Autodesk Inventor part; units mm, degrees
ref_plane "YZ Plane" through (0, 0, 0) normal (1, 0, 0) x (0, 1, 0)
ref_plane "XZ Plane" through (0, 0, 0) normal (0, 1, 0) x (-1, 0, 0)
ref_plane "XY Plane" through (0, 0, 0) normal (0, 0, 1) x (1, 0, 0)
sketch "Sketch1" plane through (0, 0, 0) normal (0, 0, 1) x (1, 0, 0)
  line L0 (0, 0) -> (25, 0)
  line L1 (25, 0) -> (25, 55.5)
  line L2 (25, 55.5) -> (0, 55.5)
  line L3 (0, 55.5) -> (0, 0)
  dimension "d0" = 25
  dimension "d1" = 55.5
extrude "Extrusion1" add sketch "Sketch1" along normal blind 3
sketch "Sketch2" plane through (0, 0, 3) normal (0, 0, 1) x (1, 0, 0)
  line L0 (0, 55.5) -> (0, 0)
  line L1 (25, 55.5) -> (0, 55.5)
  line L2 (0, 0) -> (3, 0)
  line L3 (3, 0) -> (3, 55.5)
  line L4 (3, 55.5) -> (0, 55.5)
  line L5 (0, 55.5) -> (0, 0)
  dimension "d4" = 3
extrude "Extrusion2" cut sketch "Sketch2" against normal through all
sketch "Sketch3" plane through (0, 0, 3) normal (0, 0, 1) x (1, 0, 0)
  point P0 (0, 0)
sketch "Sketch4" plane through (0, 0, 3) normal (0, 0, 1) x (1, 0, 0)
  line L0 (25, 55.5) -> (3, 55.5)
  line L1 (3, 55.5) -> (18.5, 55.5)
  line L2 (18.5, 55.5) -> (18.5, 22.5)
  line L3 (18.5, 22.5) -> (3, 22.5)
  line L4 (3, 22.5) -> (3, 55.5)
  point P0 (0, 0)
  dimension "d7" = 15.5
  dimension "d8" = 33
extrude "Extrusion3" cut sketch "Sketch4" against normal through all
sketch "Sketch5" plane through (0, 0, 3) normal (0, 0, 1) x (1, 0, 0)
  line L0 (3, 0) -> (25, 0)
  line L1 (8, 0) -> (18, 0)
  line L2 (18, 0) -> (18, 3)
  line L3 (18, 3) -> (8, 3)
  line L4 (8, 3) -> (8, 0)
  line L5 (3, 22.5) -> (3, 0)
  line L6 (3, 0) -> (8, 0)
  line L7 (8, 0) -> (8, 3)
  line L8 (8, 3) -> (3, 3)
  line L9 (3, 3) -> (3, 0)
  line L10 (18, 0) -> (25, 0)
  line L11 (25, 0) -> (25, 3)
  line L12 (25, 3) -> (18, 3)
  line L13 (18, 3) -> (18, 0)
  point P0 (0, 0)
  dimension "d11" = 10
  dimension "d12" = 3
  dimension "d13" = 5
extrude "Extrusion4" cut sketch "Sketch5" against normal through all contours L5 L8 L4 L0 | L2 L12 L11 L0
sketch "Sketch6" plane through (0, 0, 3) normal (0, 0, 1) x (1, 0, 0)
  line L0 (8, 0) -> (18, 0)
  line L1 (18, 3) -> (25, 3)
  line L2 (8, 0) -> (18, 0)
  line L3 (18, 0) -> (18, 3)
  line L4 (18, 3) -> (8, 3)
  line L5 (8, 3) -> (8, 0)
  point P0 (0, 0)
extrude "Extrusion5" cut sketch "Sketch6" against normal through all
sketch "Sketch7" plane through (0, 0, 3) normal (0, 0, 1) x (1, 0, 0)
  line L0 (3, 22.5) -> (3, 3)
  line L1 (3, 17.5) -> (0, 17.5)
  line L2 (0, 17.5) -> (0, 7.5)
  line L3 (0, 7.5) -> (3, 7.5)
  line L4 (3, 7.5) -> (3, 17.5)
  line L5 (3, 3) -> (25, 3)
  point P0 (0, 0)
  dimension "d18" = 3
  dimension "d19" = 10
  dimension "d20" = 4.5
extrude "Extrusion6" add sketch "Sketch7" against normal blind 3
properties part number "hollow_mount"
Geometry: final body of the model. Coordinates: model frame, mm. A direction names the side the tool comes from. Coordinates: 2 decimals unless noted, no trailing zeros. Order: outer loops, then holes, each group sorted by start corner. A loop starts at its lowest first (then second) coordinate and runs counter-clockwise, first axis right, second up.
1) Section C-C (x = 14). Return loops of the section in (y, z).
Result sheet:
outline: (3, 0) - (22.5, 0) - (22.5, 3) - (3, 3) - close
2) Section B-B (y = 6.5). Return loops of the section in (x, z), then the cut area to 3 significant figures.
Result sheet:
outline: (3, 0) - (25, 0) - (25, 3) - (3, 3) - close
area: 66.0 mm2
3) First-contact query: P1, Ø0.9, axis at y = 5.5, z = 2, coming from the -X side; P2, Ø1, axis at y = 41.5, z = 2.5, coming from the -X side; P3, Ø1.5, axis at x = 1.5, z = 2, coming from the -Y side. Flat tips, straight axial feed; report the tip coordinate or a pass-through.
Result sheet:
P1: stops at x = 3
P2: stops at x = 18.5
P3: stops at y = 7.5
4) Ray query, probe 1 along Y at (x, z) = (14.75, 1.9); probe 2 along X at (y, z) = (6, 0.35); probe 3 along X at (y, z) = (36.5, 0.2). Return the intervals inside material, ascending.
Result sheet:
probe 1: y = 3 to 22.5
probe 2: x = 3 to 25
probe 3: x = 18.5 to 25
5) Section A-A (z = 0.7). Return loops of the section in (x, y), then the cut area to 4 significant figures.
Result sheet:
outline: (0, 7.5) - (3, 7.5) - (3, 3) - (25, 3) - (25, 55.5) - (18.5, 55.5) - (18.5, 22.5) - (3, 22.5) - (3, 17.5) - (0, 17.5) - close
area: 673.5 mm2
6) Set-up query: faces 1 (the flat face through (1, 7.5, 2)), 2 (the flat face through (0, 13, 2)), 3 (the flat face through (18.5, 39, 2)). Return all of +Z, -Z, +X, -X, +Y, -Y with unobstructed straight access to the full face (end or side cutting, diameter ignored); none if empty.
Result sheet:
face 1: +Z, -Z, -X, -Y
face 2: +Z, -Z, -X, +Y, -Y
face 3: +Z, -Z, -X, +Y
